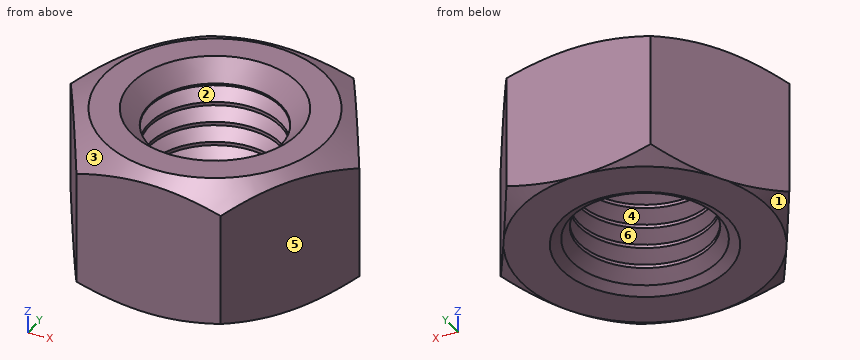
```python
from build123d import *

# Parameters (mm, degrees)
SKETCH1_R        = 3.4585
BASENUT_DEPTH    = 7.5
ENDCHAMFER2_SIZE = 0.9165
LPATTERN10_COUNT = 6
LPATTERN10_PITCH = 1.0998


with BuildPart() as part:
    # Sketch1 → BaseNut (new body)
    with BuildSketch(Plane.XY):
        Polygon((3.75277675, -6.5), (7.505553499, 0), (3.75277675, 6.5), (-3.75277675, 6.5), (-7.505553499, 0), (-3.75277675, -6.5), align=None)
        Circle(SKETCH1_R, mode=Mode.SUBTRACT)
    extrude(amount=-BASENUT_DEPTH)

    # Sketch2 → Chamfer1 (revolve, cut)
    with BuildSketch(Plane(origin=(15.04811501, 0, -16.706149795), x_dir=(0, 0, -1), z_dir=(0, 1, 0))):
        Polygon((-9.786706379, 22.553668509), (-9.206149795, 21.54811501), (-9.206149795, 22.553668509), align=None)
    revolve(axis=Axis((0, 0, 7.016501752), (0, 0, -1)), mode=Mode.SUBTRACT)

    # Sketch6 → EndChamfer1 (revolve, cut)
    with BuildSketch(Plane(origin=(-9.197458863, 0, -10.252541137), x_dir=(0, 0, 1), z_dir=(0, 1, 0))):
        Polygon((2.752541137, 12.655958863), (2.752541137, 13.572458863), (3.281682659, 12.655958863), align=None)
    revolve(axis=Axis((0, 0, 13.104863586), (0, 0, -1)), mode=Mode.SUBTRACT)

    # Sketch5 → Chamfer2 (revolve, cut)
    with BuildSketch(Plane(origin=(-14.793032735, 0, -16.96123207), x_dir=(0, 0, 1), z_dir=(0, 1, 0))):
        Polygon((16.96123207, 20.608032735), (16.96123207, 22.298586235), (15.985190552, 22.298586235), align=None)
    revolve(axis=Axis((0, 0, -39.536013381), (0, 0, 1)), mode=Mode.SUBTRACT)

    # EndChamfer2
    endchamfer2_edges = [part.edges().sort_by_distance(p)[0] for p in [
        (-3.4585, 0, 0),
    ]]
    chamfer(endchamfer2_edges, length=ENDCHAMFER2_SIZE)

    # Sketch7 → Cut-Revolve10 (revolve, cut)
    with BuildSketch(Plane(origin=(0, 0, 0), x_dir=(1, 0, 0), z_dir=(0, 1, 0))):
        Polygon((2.542, 7.429108478), (3.4585, 7.429108478), (4.252212283, 6.970858478), (3.4585, 6.512608478), (2.542, 6.512608478), align=None)
    cut_revolve10 = revolve(axis=Axis((0, 0, -48.618332322), (0, 0, 1)), mode=Mode.SUBTRACT)

    # LPattern10: Cut-Revolve10 ×6
    with Locations(*[(0, 0, i * LPATTERN10_PITCH) for i in range(1, LPATTERN10_COUNT)]):
        add(cut_revolve10, mode=Mode.SUBTRACT)


solid = part.part
```
Geometry: final body of the model. Coordinates: model frame, mm. Face numbers are marked on the shaded views. A direction names the side the tool comes from. Round coordinates to 2 decimals unless told otherwise and drop trailing zeros. Order: outer loops, then holes, each group sorted by start corner. A loop starts at its lowest first (then second) coordinate and runs counter-clockwise, first axis right, second up. Notation, with made-up numbers: (62, 78) -> (112, 78) arc R4 ccw to (112, 83) -> close; hole circle Ø10 at (-36.5, -28.75). An arc over 180 degrees is marked (long way). Use CSV: the item, a comma, the result in double quotes. Start each with the question number.
1) Material intervals for line 1 along X through (y, z) = (1.75, -2.25); line 2 along X through (y, z) = (-1, -2.75); line 3 along Y through (x, z) = (0, -0.95), sorted ascending. Write a range as from..to.
2) First-contact query: pin 1 Ø5.5 at (x, y) = (0, 0) entering from +Z; pin 2 Ø1 at (y, z) = (3, -6.5) entering from +X; pin 3 Ø6 at (x, y) = (-0.5, -0.5) entering from +Z; pin 4 Ø4 at (x, z) = (6, -6) entering from +Y. Flat tips, straight axial feed; report the tip coordinate or a pass-through.
3) Section A-A (z = -1.75). Return the cut outline in (x, y).
4) Set-up query: the marked faces 5 and 6. Return all of +Z, -Z, +X, -X, +Y, -Y with unobstructed straight access to the full face (end or side cutting, diameter ignored); none if empty.
5) Draft query along Z for the marked faces 1, 2, 3 and 4. Return one class per face: +Z half, -Z half, draft (parallel to the pull), parting line (faces both ways), or undercut.
6) Section B-B (z = -4.5). Return the cut outline in (x, y), and give its area (3 significant figures).
Returned:
1,line 1,"x = -6.5..-3.25, 3.25..6.5"
1,line 2,"x = -6.93..-3.81, 3.81..6.93"
1,line 3,"y = -6.5..-3.46, 3.46..6.5"
2,pin 1,"passes through"
2,pin 2,"stops at x = 6.06"
2,pin 3,"stops at z = -0.67"
2,pin 4,"stops at y = 6.07"
3,outline,"(-7.51, 0) -> (-3.75, -6.5) -> (3.75, -6.5) -> (7.51, 0) -> (3.75, 6.5) -> (-3.75, 6.5) -> close; hole circle Ø7.54 at (0, 0)"
4,face 5,"+Z, -Z, +X, -Y"
4,face 6,"none"
5,face 1,"-Z half"
5,face 2,"undercut"
5,face 3,"+Z half"
5,face 4,"undercut"
6,outline,"(-7.51, 0) -> (-3.75, -6.5) -> (3.75, -6.5) -> (7.51, 0) -> (3.75, 6.5) -> (-3.75, 6.5) -> close; hole circle Ø7.56 at (0, 0)"
6,area,"101 mm²"
